Design review of the part built by this model. Coordinates are the model's own, in mm. A direction names the side the tool comes from. Coordinates: 2 decimals unless noted, no trailing zeros. Loops run counter-clockwise (first coordinate to the right, second up) from the corner with the lowest first, then second, coordinate; pieces in that order, holes last.
Q1. Add section B-B on y = -74. Give the boundary of the cut face in (x, z).
Q2. Wall thickness on probe 1 along X at (y, z) = (-45.5, 0.5); probe 2 along Y at (x, z) = (33, 4.55); probe 3 along X at (y, z) = (-38.5, 3.8): over which ranges is each line inside the solid? List them lowest first.
Q3. Add section C-C on z = 0.8. Give the boundary of the cut face in (x, y).
Q4. Add section A-A on x = 7. Give the boundary of the cut face in (y, z).
Q5. Draft analysis for pull direction Y (two halves, no side actions). For faces 5 (the face through (39.01, 0.91, 2.46)), 6 (the face through (75, -22, 0)), 7 (the face through (62.762, -58, 2)), state which applies: released by +Y, released by -Y, zero draft, split by the parting line, or undercut.
Q6. For P1, Ø1.4, axis at x = 47.5, z = 2, coming from the -Y side; P2, Ø2.5, axis at y = -54, z = 2.5, coming from the +X side; P3, Ø1.5, axis at y = -61, z = 1.5, coming from the -X side; P4, Ø3, axis at x = 136.5, y = -27.5, coming from the -Z side, all flat-tipped, find the tip position at first contact; note any pin that passes through.
Q7. Add section D-D on x = 71.5. Give the boundary of the cut face in (y, z).
Q8. Machinability: for faces 1 (the face through (6, -14.994, 2)), 2 (the face through (122, -17.214, 2)), 3 (the face through (13, 0, 2)), 4 (the face through (66.762, -57, 2)), which of the approach directions +Z, -Z, +X, -X, +Y, -Y give a long, thin tool a straight path to every point of the face, cutting with its end or side? Answer none if there is none.
Autodesk Inventor part; units mm, degrees
ref_plane "YZ Plane" through (0, 0, 0) normal (1, 0, 0) x (0, 1, 0)
ref_plane "XZ Plane" through (0, 0, 0) normal (0, 1, 0) x (-1, 0, 0)
ref_plane "XY Plane" through (0, 0, 0) normal (0, 0, 1) x (1, 0, 0)
sketch "Boceto1" plane through (0, 0, 0) normal (0, 0, 1) x (1, 0, 0)
  circle A0 centre (7, -5) radius 3.5
  arc A1 (66.7617, -38.7297) -> (62.7617, -38.7297) centre (64.7617, -38.7297) ccw
  line L0 (66.7617, -38.7297) -> (66.7617, -75.9094)
  arc A2 (62.7617, -75.9094) -> (66.7617, -75.9094) centre (64.7617, -75.9094) ccw
  line L1 (62.7617, -75.9094) -> (62.7617, -38.7297)
  line L2 (163.1909, -24.7137) -> (163.1909, -17.2137)
  line L3 (163.1909, -17.2137) -> (79.2209, -17.2137)
  arc A3 (76.5087, -16.8389) -> (79.2209, -17.2137) centre (79.2209, -7.2137) ccw
  line L4 (76.5087, -16.8389) -> (52.321, -10.0234)
  arc A4 (52.321, -10.0234) -> (50.4155, -9.6811) centre (49.6089, -19.6486) ccw
  arc A5 (48.4983, -9.3356) -> (50.4155, -9.6811) centre (51.2221, 0.2863) ccw
  arc A6 (17.4207, -16.6942) -> (45.0673, -24.7137) centre (33.1909, -13.9922) ccw
  line L5 (45.0673, -24.7137) -> (49.8402, -24.7137)
  arc A7 (52.5523, -25.0885) -> (49.8402, -24.7137) centre (49.8402, -34.7137) ccw
  line L6 (52.5523, -25.0885) -> (60.7617, -27.4017)
  line L7 (60.7617, -27.4017) -> (60.7617, -79.4017)
  arc A8 (60.7617, -79.4017) -> (68.7617, -79.4017) centre (64.7617, -79.6579) ccw
  line L8 (68.7617, -79.4017) -> (68.7617, -29.656)
  line L9 (68.7617, -29.656) -> (76.5087, -31.8389)
  arc A9 (76.5087, -31.8389) -> (79.2209, -32.2137) centre (79.2209, -22.2137) ccw
  line L10 (79.2209, -32.2137) -> (163.1909, -32.2137)
  line L11 (163.1909, -32.2137) -> (163.1909, -17.2137)
  line L12 (25.4308, 0) -> (0, 0)
  line L13 (0, 0) -> (0, -14.9941)
  line L14 (0, -14.9941) -> (11.843, -14.9941)
  arc A10 (17.4207, -16.6942) -> (11.843, -14.9941) centre (11.843, -24.9941) ccw
  arc A11 (48.4983, -9.3356) -> (25.4308, 0) centre (33.1909, -13.9922) ccw
  circle A12 centre (33.1909, -13.9922) radius 1
  point P0 (52.321, -10.0234)
  point P1 (50.4155, -9.6811)
  point P2 (48.4983, -9.3356)
  point P3 (11.843, -14.9941)
  point P4 (17.4207, -16.6942)
  point P5 (45.0673, -24.7137)
  point P6 (49.8402, -24.7137)
  point P7 (52.5523, -25.0885)
  point P8 (60.7617, -79.4017)
  point P9 (68.7617, -79.4017)
  point P10 (79.2209, -32.2137)
  dimension "d0" = 2
extrude "Extrusión1" add sketch "Boceto1" along normal blind 5
properties part number "P6"
Entries:
1. outline: (60.76, 0) - (62.76, 0) - (62.76, 5) - (60.76, 5) - close; (66.76, 0) - (68.76, 0) - (68.76, 5) - (66.76, 5) - close
2. probe 1: x = 60.76 to 62.76, 66.76 to 68.76
2. probe 2: y = -29.99 to -14.97, -13.01 to 2.01
2. probe 3: x = 60.76 to 62.77, 66.75 to 68.76
3. outline: (0, -14.99) - (11.84, -14.99) arc R10 cw to (17.42, -16.69) arc R16 ccw to (45.07, -24.71) - (49.84, -24.71) arc R10 cw to (52.55, -25.09) - (60.76, -27.4) - (60.76, -79.4) arc R4.01 ccw (long way) to (68.76, -79.4) - (68.76, -29.66) - (76.51, -31.84) arc R10 ccw to (79.22, -32.21) - (163.19, -32.21) - (163.19, -17.21) - (79.22, -17.21) arc R10 cw to (76.51, -16.84) - (52.32, -10.02) arc R10.01 ccw to (50.42, -9.68) arc R10 cw to (48.5, -9.34) arc R16 ccw to (25.43, 0) - (0, 0) - close; hole circle Ø7 at (7, -5); hole circle Ø2 at (33.19, -13.99); hole (62.76, -75.91) arc R2 ccw to (66.76, -75.91) - (66.76, -38.73) arc R2 ccw to (62.76, -38.73) - close
4. outline: (-14.99, 0) - (-8.5, 0) - (-8.5, 5) - (-14.99, 5) - close; (-1.5, 0) - (0, 0) - (0, 5) - (-1.5, 5) - close
5. face 5: released by +Y
5. face 6: zero draft
5. face 7: undercut
6. P1: stops at y = -24.71
6. P2: stops at x = 68.76
6. P3: stops at x = 60.76
6. P4: stops at z = 0
7. outline: (-30.43, 0) - (-15.43, 0) - (-15.43, 5) - (-30.43, 5) - close
8. face 1: +Z, -Z, -X, -Y
8. face 2: +Z, -Z, +X, +Y
8. face 3: +Z, -Z, -X, +Y
8. face 4: +Z, -Z
